from build123d import *

# Parameters (mm, degrees)
F2_W          = 9
F2_H          = 12.5
F3_DEPTH      = 18.5
F4_W          = 4
F4_H          = 4
F5_DEPTH      = 2.5
F6_R          = 2
F7_DEPTH      = 16.751
F7_DEPTH_BACK = 16.751


with BuildPart() as f1:
    # F0 (on Front) → F1 (revolve)
    with BuildSketch(Plane.XZ):
        Polygon((0, 18.5), (0, 0), (16.75, 0), (16.75, 2.5), (11.5, 2.5), (11.5, 15.5), (8.75, 15.5), (8.75, 18.5), align=None)
    revolve(axis=Axis((0, 0, 44.9704285987), (0, 0, 1)))

    # F2 (on face) → F3 (cut, through all)
    with BuildSketch(Plane.XY.offset(18.5)):
        Rectangle(F2_W, F2_H)
    extrude(amount=-F3_DEPTH, mode=Mode.SUBTRACT)

    # F4 (on face) → F5 (join)
    with BuildSketch(Plane(origin=(0, 0, 0), x_dir=(1, 0, 0), z_dir=(0, 0, -1))):
        with Locations((1.5, 8.75)):
            Rectangle(F4_W, F4_H)
    extrude(amount=F5_DEPTH)

    # F6 (on Right) → F7 (cut, two sides)
    with BuildSketch(Plane.YZ) as f7_sk:
        with Locations((0, 9.5)):
            Circle(F6_R)
    extrude(amount=-F7_DEPTH, mode=Mode.SUBTRACT)
    extrude(f7_sk.sketch, amount=F7_DEPTH_BACK, mode=Mode.SUBTRACT)


solid = f1.part
Geometry check sheet. Reference: the model listing, model coordinates, mm. A direction names the side the tool comes from. Round coordinates to 2 decimals unless told otherwise and drop trailing zeros. Order: outer loops, then holes, each group sorted by start corner. A loop starts at its lowest first (then second) coordinate and runs counter-clockwise, first axis right, second up. Notation, with made-up numbers: (81.25, -8.75) -> (109.25, -8.75) arc R11 ccw to (109.25, 1.25) -> close; hole circle Ø5 at (42.5, 63). An arc over 180 degrees is marked (long way). Use one line per item in the form item = value.
1. Go/stop test with flat-tipped pins: pin 1 (3 mm diameter, centred on y = -9.5, z = 8, fed in from -X); pin 2 (6 mm diameter, centred on y = -2.5, z = 7, fed in from -X); pin 3 (1.2 mm diameter, centred on x = 2.5, z = -1.5, fed in from -Y). Record where each tip stops, or that it passes through.
Working result:
pin_1 = -8.26
pin_2 = -11.5
pin_3 = -10.75
2. Cross-section at C-C, the plane z = 9.5. Enter the section's corners in (x, y), plus the area to 3 significant figures.
Working result:
outline = (-11.32, -2) arc R11.5 ccw to (11.32, -2) -> (4.5, -2) -> (4.5, -6.25) -> (-4.5, -6.25) -> (-4.5, -2) -> close; (-11.32, 2) -> (-4.5, 2) -> (-4.5, 6.25) -> (4.5, 6.25) -> (4.5, 2) -> (11.32, 2) arc R11.5 ccw to start
area = 247 mm^2
3. Set-up check for faces 4 (the face through (1, -6.75, -1)), 5 (the face through (1, -10.75, -1)), 6 (the face through (-0.5, -9, -1)), 7 (the face through (-6.944, -5.324, 17.021)), 8 (the face through (0, 6.25, 9)): record each of +Z, -Z, +X, -X, +Y, -Y from which the full face is reachable in a straight line by a thin tool's end or side.
Working result:
face_4 = -Z, +X, -X, +Y
face_5 = -Z, +X, -X, -Y
face_6 = -Z, -X, +Y, -Y
face_7 = +Z
face_8 = +Z, -Z
4. Mould release check, pull along Z, two halves, no side actions. Record for faces 1 (the face through (-3.63, -16.35, 1.27)), 2 (the face through (-4, -11, 2.5)), 3 (the face through (-7.953, -0.26, 11.483)): pulls with the +Z half, pulls with the -Z half, needs draft (parallel to the pull), parting line crosses it, or undercut.
Working result:
face_1 = needs draft
face_2 = pulls with the +Z half
face_3 = undercut
5. Cross-section at D-D, the plane z = 12.75. Enter the section's corners in (x, y).
Working result:
outline = circle Ø23 at (0, 0); hole (-4.5, -6.25) -> (4.5, -6.25) -> (4.5, 6.25) -> (-4.5, 6.25) -> close
6. Cross-section at A-A, the plane y = 0. Enter the section's corners in (x, z), plus the area to 3 significant figures.
Working result:
outline = (-16.75, 0) -> (-4.5, 0) -> (-4.5, 7.5) -> (-11.5, 7.5) -> (-11.5, 2.5) -> (-16.75, 2.5) -> close; (-11.5, 11.5) -> (-4.5, 11.5) -> (-4.5, 18.5) -> (-8.75, 18.5) -> (-8.75, 15.5) -> (-11.5, 15.5) -> close; (4.5, 0) -> (16.75, 0) -> (16.75, 2.5) -> (11.5, 2.5) -> (11.5, 7.5) -> (4.5, 7.5) -> close; (4.5, 11.5) -> (11.5, 11.5) -> (11.5, 15.5) -> (8.75, 15.5) -> (8.75, 18.5) -> (4.5, 18.5) -> close
area = 213 mm^2
7. Scan lines: line 1 along Z through (x, y) = (8, 0); line 2 along Z through (x, y) = (5.5, 8.5); line 3 along X through (y, z) = (5.5, 7.25). Record each from-to range of solid material in increasing order. Write a range as from..to.
Working result:
line_1 = 0..7.5, 11.5..18.5
line_2 = 0..15.5
line_3 = -10.1..-4.5, 4.5..10.1
8. Cross-section at B-B, the plane x = 0. Enter the section's corners in (y, z), plus the area to 3 significant figures.
Working result:
outline = (-16.75, 0) -> (-10.75, 0) -> (-10.75, -2.5) -> (-6.75, -2.5) -> (-6.75, 0) -> (-6.25, 0) -> (-6.25, 18.5) -> (-8.75, 18.5) -> (-8.75, 15.5) -> (-11.5, 15.5) -> (-11.5, 2.5) -> (-16.75, 2.5) -> close; (6.25, 0) -> (16.75, 0) -> (16.75, 2.5) -> (11.5, 2.5) -> (11.5, 15.5) -> (8.75, 15.5) -> (8.75, 18.5) -> (6.25, 18.5) -> close
area = 214 mm^2
